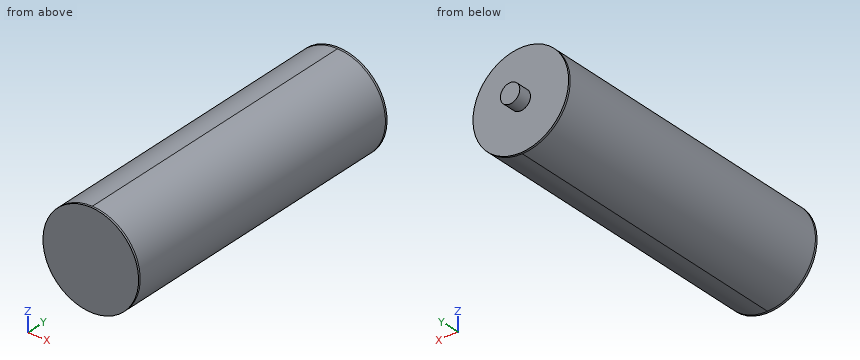
```python
from build123d import *
from build123d.topology import SkipClean

# Parameters (mm, degrees)
SKETCH1_R           = 7.25
BOSS_EXTRUDE1_DEPTH = 46
SKETCH2_R           = 7
CUT_EXTRUDE1_DEPTH  = 64.5
SKETCH4_R           = 7.25
BOSS_EXTRUDE2_DEPTH = 46
SKETCH6_R           = 1.471316345
BOSS_EXTRUDE3_DEPTH = 2


with BuildPart() as part:
    # Sketch1 → Boss-Extrude1 (new body)
    with BuildSketch(Plane(origin=(0, 0, 0), x_dir=(1, 0, 0), z_dir=(0, 1, 0))):
        with Locations(Location((0, 0, 0), (0, 0, 270))):
            Circle(SKETCH1_R)
    extrude(amount=BOSS_EXTRUDE1_DEPTH)

    # Sketch2 → Cut-Extrude1 (cut)
    with BuildSketch(Plane(origin=(0, 0.3, 0), x_dir=(-1, 0, 0), z_dir=(0, -1, 0))):
        with Locations(Location((0, 0, 0), (0, 0, 90))):
            Circle(SKETCH2_R)
    extrude(amount=-CUT_EXTRUDE1_DEPTH, mode=Mode.SUBTRACT)

    # Sketch4 → Boss-Extrude2 (add)
    with SkipClean():  # the faces are left unmerged after this step: merging them gives an invalid solid
        with BuildSketch(Plane(origin=(0, 0.3, 0), x_dir=(-1, 0, 0), z_dir=(0, -1, 0))):
            with Locations(Location((0, 0, 0), (0, 0, 90))):
                Circle(SKETCH4_R)
        extrude(amount=-BOSS_EXTRUDE2_DEPTH)
    add(part.part.scale(1), mode=Mode.REPLACE)  # the faces are merged on a copy

    # Sketch6 → Boss-Extrude3 (add)
    with BuildSketch(Plane(origin=(0, 46.3, 0), x_dir=(1, 0, 0), z_dir=(0, 1, 0))):
        with Locations(Location((0, 0, 0), (0, 0, 270))):
            Circle(SKETCH6_R)
    extrude(amount=BOSS_EXTRUDE3_DEPTH)


solid = part.part
```
Part model, mm, in its own coordinate system. Round coordinates to 2 decimals unless told otherwise and drop trailing zeros. Loops run counter-clockwise (first coordinate to the right, second up) from the corner with the lowest first, then second, coordinate; pieces in that order, holes last.
1. Slice it at A-A (x = 0.75). Give the cut face in (y, z), and give its area (3 significant figures).
Solutions:
outline: (0, -7.21) - (46.3, -7.21) - (46.3, -1.27) - (48.3, -1.27) - (48.3, 1.27) - (46.3, 1.27) - (46.3, 7.21) - (0, 7.21) - close
area: 673 mm2
2. Slice it at C-C (y = 32.5). Give the cut face in (x, z), and give its area (3 significant figures).
Solutions:
outline: circle Ø14.5 at (0, 0)
area: 165 mm2
3. Drill centre lines: line 1 along Y through (x, z) = (2.5, 2); line 2 along Z through (x, y) = (1, 24.5); line 3 along X through (y, z) = (44.5, -4). Where is each one in solid material? Low to high.
Solutions:
line 1: y = 0 to 46.3
line 2: z = -7.18 to 7.18
line 3: x = -6.05 to 6.05
4. Flat gauge pins, fed straight in: pin 1 (2 mm diameter, centred on y = 26.5, z = -1.5, fed in from -X); pin 2 (3 mm diameter, centred on y = 24.5, z = -4, fed in from +X); pin 3 (2 mm diameter, centred on y = 13, z = 5, fed in from +X). Where does each tip first touch, or does it go through?
Solutions:
pin 1: stops at x = -7.23
pin 2: stops at x = 6.81
pin 3: stops at x = 6.05
5. Slice it at D-D (z = -2). Give the cut face in (x, y), and give its area (3 significant figures).
Solutions:
outline: (-6.97, 0) - (6.97, 0) - (6.97, 46.3) - (-6.97, 46.3) - close
area: 645 mm2
6. Slice it at B-B (z = 0). Give the cut face in (x, y).
Solutions:
outline: (-7.25, 0) - (7.25, 0) - (7.25, 46.3) - (1.47, 46.3) - (1.47, 48.3) - (-1.47, 48.3) - (-1.47, 46.3) - (-7.25, 46.3) - close
